Geometry check sheet. Reference: the model listing, model coordinates, mm. A direction names the side the tool comes from. Give positions to 0.01 mm unless a question says otherwise; leave off trailing zeros. Order: outer loops, then holes, each group sorted by start corner. A loop starts at its lowest first (then second) coordinate and runs counter-clockwise, first axis right, second up. Notation, with made-up numbers: M -3.75,50 L 13.25,50 A20 cw 13.25,58 Z; hole C 4,14.5 d8. An arc over 180 degrees is marked long. Answer as a JSON object with one key per item and string values. Group by question number.
from build123d import *

# Parameters (mm, degrees)
SKETCH7_R             = 4.411628617
SKETCH7_R_2           = 1.499999999
BOSS_EXTRUDE1_DEPTH   = 15
SKETCH7_R_3           = 4.404719082
BOSS_EXTRUDE1_2_DEPTH = 15
BOSS_EXTRUDE1_3_DEPTH = 15
BOSS_EXTRUDE1_4_DEPTH = 15
SKETCH8_R             = 3.5
CUT_EXTRUDE1_DEPTH    = 5
SKETCH9_R             = 3.5
BOSS_EXTRUDE9_DEPTH   = 5
SKETCH12_R            = 2.1
BOSS_EXTRUDE10_DEPTH  = 5
FILLET3_R             = 4
SKETCH13_W            = 20
SKETCH13_H            = 20
SKETCH13_R            = 2.383284349
BOSS_EXTRUDE11_DEPTH  = 5
FILLET4_R             = 4
SKETCH14_R            = 2.383284349
SKETCH14_R_2          = 2.1
SKETCH14_W            = 20
SKETCH14_H            = 40
BOSS_EXTRUDE12_DEPTH  = 5
FILLET5_R             = 4
SKETCH15_W            = 31.82070186
SKETCH15_H            = 40
SKETCH15_R            = 2.1
BOSS_EXTRUDE13_DEPTH  = 5
FILLET6_R             = 4
SKETCH16_R            = 3.5
SKETCH16_R_2          = 1.499999999
BOSS_EXTRUDE14_DEPTH  = 15
CUT_EXTRUDE3_DEPTH    = 15
SKETCH18_R            = 13.5
CUT_EXTRUDE6_DEPTH    = 21


with BuildPart() as part:
    # Sketch7 → Boss-Extrude1 (new body)
    with BuildSketch(Plane(origin=(0, 0, 0), x_dir=(1, 0, 0), z_dir=(0, 1, 0))):
        with Locations((-35.224970632, 25)):
            Circle(SKETCH7_R)
        with Locations((-35.224970632, 25)):
            Circle(SKETCH7_R_2, mode=Mode.SUBTRACT)
    extrude(amount=-BOSS_EXTRUDE1_DEPTH)


with BuildPart() as body_2:
    # Sketch7 → Boss-Extrude1 2 (new body)
    with BuildSketch(Plane(origin=(0, 0, 0), x_dir=(1, 0, 0), z_dir=(0, 1, 0))):
        with Locations((21.775029368, 31)):
            Circle(SKETCH7_R_3)
        with Locations((21.775029368, 31)):
            Circle(SKETCH7_R_2, mode=Mode.SUBTRACT)
    extrude(amount=-BOSS_EXTRUDE1_2_DEPTH)


with BuildPart() as body_3:
    # Sketch7 → Boss-Extrude1 3 (new body)
    with BuildSketch(Plane(origin=(0, 0, 0), x_dir=(1, 0, 0), z_dir=(0, 1, 0))):
        with Locations((21.775029368, -31)):
            Circle(SKETCH7_R_3)
        with Locations((21.775029368, -31)):
            Circle(SKETCH7_R_2, mode=Mode.SUBTRACT)
    extrude(amount=-BOSS_EXTRUDE1_3_DEPTH)


with BuildPart() as body_4:
    # Sketch7 → Boss-Extrude1 4 (new body)
    with BuildSketch(Plane(origin=(0, 0, 0), x_dir=(1, 0, 0), z_dir=(0, 1, 0))):
        with Locations((-35.224970632, -25)):
            Circle(SKETCH7_R)
        with Locations((-35.224970632, -25)):
            Circle(SKETCH7_R_2, mode=Mode.SUBTRACT)
    extrude(amount=-BOSS_EXTRUDE1_4_DEPTH)


with BuildPart() as cut_extrude1_tool:
    # Sketch8 → Cut-Extrude1 (new body)
    with BuildSketch(Plane(origin=(0, -15, 0), x_dir=(-1, 0, 0), z_dir=(0, -1, 0))):
        with Locations((35.224970632, -25)):
            Circle(SKETCH8_R)
        with Locations((-21.775029368, -31)):
            Circle(SKETCH8_R)
        with Locations((35.224970632, 25)):
            Circle(SKETCH8_R)
        with Locations((-21.775029368, 31)):
            Circle(SKETCH8_R)
    extrude(amount=-CUT_EXTRUDE1_DEPTH)


with BuildPart() as part_1:
    add(part.part)

    # Cut-Extrude1: cut by cut_extrude1_tool
    add(cut_extrude1_tool.part, mode=Mode.SUBTRACT)



with BuildPart() as body_2_1:
    add(body_2.part)

    # Cut-Extrude1: cut by cut_extrude1_tool
    add(cut_extrude1_tool.part, mode=Mode.SUBTRACT)


with BuildPart() as body_3_1:
    add(body_3.part)

    # Cut-Extrude1: cut by cut_extrude1_tool
    add(cut_extrude1_tool.part, mode=Mode.SUBTRACT)


with BuildPart() as body_4_1:
    add(body_4.part)

    # Cut-Extrude1: cut by cut_extrude1_tool
    add(cut_extrude1_tool.part, mode=Mode.SUBTRACT)


with BuildPart() as part_2:
    add(part_1.part)

    add(body_2_1.part)  # Boss-Extrude9 merges body 2

    add(body_3_1.part)  # Boss-Extrude9 merges body 3

    add(body_4_1.part)  # Boss-Extrude9 merges body 4
    # Sketch9 → Boss-Extrude9 (add)
    with BuildSketch(Plane(origin=(0, -15, 0), x_dir=(-1, 0, 0), z_dir=(0, -1, 0))):
        with BuildLine():
            Line((38.764660529, -27.633070923), (55.562895144, -8.838834765))
            ThreePointArc((55.562895144, -8.838834765), (59.224060379, 0), (55.562895144, 8.838834765))
            Line((55.562895144, 8.838834765), (38.764660529, 27.633070923))
            ThreePointArc((38.764660529, 27.633070923), (37.205669501, 28.941991761), (35.224970632, 29.411628617))
            Line((35.224970632, 29.411628617), (-20.858915448, 35.308397089))
            Line((-20.858915448, 35.308397089), (-21.775029368, 35.404719082))
            ThreePointArc((-21.775029368, 35.404719082), (-24.985189946, 34.016027065), (-26.171192213, 30.725587114))
            ThreePointArc((-26.171192213, 30.725587114), (-33.931933496, 0), (-26.171192213, -30.725587114))
            ThreePointArc((-26.171192213, -30.725587114), (-24.985189946, -34.016027065), (-21.775029368, -35.404719082))
            Line((-21.775029368, -35.404719082), (-20.858915448, -35.308397089))
            Line((-20.858915448, -35.308397089), (35.224970632, -29.411628617))
            ThreePointArc((35.224970632, -29.411628617), (37.205669501, -28.941991761), (38.764660529, -27.633070923))
        make_face()
        with Locations((-21.775029368, -31)):
            Circle(SKETCH9_R, mode=Mode.SUBTRACT)
        with Locations((35.224970632, -25)):
            Circle(SKETCH9_R, mode=Mode.SUBTRACT)
        with Locations((-21.775029368, 31)):
            Circle(SKETCH9_R, mode=Mode.SUBTRACT)
        with Locations((35.224970632, 25)):
            Circle(SKETCH9_R, mode=Mode.SUBTRACT)
    extrude(amount=BOSS_EXTRUDE9_DEPTH)

    # Sketch12 → Boss-Extrude10 (add)
    with BuildSketch(Plane(origin=(0, -15, 0), x_dir=(1, 0, 0), z_dir=(0, 1, 0))):
        Polygon((0, 29.508444845), (15.196340386, 29.508444845), (15.196340386, 44.508444845), (-20, 44.508444845), (-20, 29.508444845), (-15, 29.508444845), align=None)
        with Locations((-15, 39.200262185)):
            Circle(SKETCH12_R, mode=Mode.SUBTRACT)
        with Locations((10.196340386, 39.200262185)):
            Circle(SKETCH12_R, mode=Mode.SUBTRACT)
        Polygon((-20, -44.508444845), (-20, -29.508444845), (-15, -29.508444845), (0, -29.508444845), (15.196340386, -29.508444845), (15.196340386, -44.508444845), align=None)
        with Locations((-15, -39.200262185)):
            Circle(SKETCH12_R, mode=Mode.SUBTRACT)
        with Locations((10.196340386, -39.200262185)):
            Circle(SKETCH12_R, mode=Mode.SUBTRACT)
    extrude(amount=-BOSS_EXTRUDE10_DEPTH)

    # Fillet3
    fillet3_edges = [part_2.edges().sort_by_distance(p)[0] for p in [
        (15.196340386, -17.5, 44.508444845),
        (-20, -17.5, 44.508444845),
        (15.196340386, -17.5, -44.508444845),
        (-20, -17.5, -44.508444845),
    ]]
    fillet(fillet3_edges, radius=FILLET3_R)

    # Sketch13 → Boss-Extrude11 (add)
    with BuildSketch(Plane(origin=(0, -15, 0), x_dir=(1, 0, 0), z_dir=(0, 1, 0))):
        with Locations((-60.435748909, 0)):
            Rectangle(SKETCH13_W, SKETCH13_H)
        with Locations((-65.435748909, 5)):
            Circle(SKETCH13_R, mode=Mode.SUBTRACT)
        with Locations((-65.435748909, -5)):
            Circle(SKETCH13_R, mode=Mode.SUBTRACT)
    extrude(amount=-BOSS_EXTRUDE11_DEPTH)

    # Fillet4
    fillet4_edges = [part_2.edges().sort_by_distance(p)[0] for p in [
        (-70.435748909, -17.5, -10),
        (-70.435748909, -17.5, 10),
    ]]
    fillet(fillet4_edges, radius=FILLET4_R)

    # Sketch14 → Boss-Extrude12 (add)
    with BuildSketch(Plane(origin=(0, -15, 0), x_dir=(1, 0, 0), z_dir=(0, 1, 0))):
        with Locations((-65.435748909, 5)):
            Circle(SKETCH14_R)
        with Locations((-65.435748909, 5)):
            Circle(SKETCH14_R_2, mode=Mode.SUBTRACT)
        with Locations((-65.435748909, -5)):
            Circle(SKETCH14_R)
        with Locations((-65.435748909, -5)):
            Circle(SKETCH14_R_2, mode=Mode.SUBTRACT)
        with Locations((33.931933496, 0)):
            Rectangle(SKETCH14_W, SKETCH14_H)
        with Locations((38.931933496, 15)):
            Circle(SKETCH14_R_2, mode=Mode.SUBTRACT)
        with Locations((38.931933496, -15)):
            Circle(SKETCH14_R_2, mode=Mode.SUBTRACT)
    extrude(amount=-BOSS_EXTRUDE12_DEPTH)

    # Fillet5
    fillet5_edges = [part_2.edges().sort_by_distance(p)[0] for p in [
        (43.931933496, -17.5, -20),
        (43.931933496, -17.5, 20),
    ]]
    fillet(fillet5_edges, radius=FILLET5_R)

    # Sketch15 → Boss-Extrude13 (add)
    with BuildSketch(Plane(origin=(0, -15, 0), x_dir=(1, 0, 0), z_dir=(0, 1, 0))):
        with Locations((-54.525048972, 0)):
            Rectangle(SKETCH15_W, SKETCH15_H)
        with Locations((-65.435748909, 15)):
            Circle(SKETCH15_R, mode=Mode.SUBTRACT)
        with Locations((-65.435748909, -15)):
            Circle(SKETCH15_R, mode=Mode.SUBTRACT)
    extrude(amount=-BOSS_EXTRUDE13_DEPTH)

    # Fillet6
    fillet6_edges = [part_2.edges().sort_by_distance(p)[0] for p in [
        (-70.435399902, -17.5, -20),
        (-70.435399902, -17.5, 20),
    ]]
    fillet(fillet6_edges, radius=FILLET6_R)

    # Sketch16 → Boss-Extrude14 (add)
    with BuildSketch(Plane(origin=(0, -20, 0), x_dir=(-1, 0, 0), z_dir=(0, -1, 0))):
        with Locations((-21.775029368, -31)):
            Circle(SKETCH16_R)
        with Locations((-21.775029368, -31)):
            Circle(SKETCH16_R_2, mode=Mode.SUBTRACT)
        with Locations((-21.775029368, 31)):
            Circle(SKETCH16_R)
        with Locations((-21.775029368, 31)):
            Circle(SKETCH16_R_2, mode=Mode.SUBTRACT)
        with Locations((35.224970632, 25)):
            Circle(SKETCH16_R)
        with Locations((35.224970632, 25)):
            Circle(SKETCH16_R_2, mode=Mode.SUBTRACT)
        with Locations((35.224970632, -25)):
            Circle(SKETCH16_R)
        with Locations((35.224970632, -25)):
            Circle(SKETCH16_R_2, mode=Mode.SUBTRACT)
    extrude(amount=-BOSS_EXTRUDE14_DEPTH)

    # Sketch17 → Cut-Extrude3 (cut)
    with BuildSketch(Plane(origin=(0, -15, 0), x_dir=(1, 0, 0), z_dir=(0, 1, 0))):
        Polygon((-30.224970632, 15), (16.775029368, 20), (16.775029368, -20), (-30.224970632, -15), align=None)
    extrude(amount=-CUT_EXTRUDE3_DEPTH, mode=Mode.SUBTRACT)

    # Sketch18 → Cut-Extrude6 (cut, through all)
    with BuildSketch(Plane(origin=(0, 0, 0), x_dir=(1, 0, 0), z_dir=(0, 1, 0))):
        with Locations((-46.724970632, 0)):
            Circle(SKETCH18_R)
    extrude(amount=-CUT_EXTRUDE6_DEPTH, mode=Mode.SUBTRACT)


solid = part_2.part
1. Cross-section at C-C (z = -25). Record the cut outline in (x, y), and give its area (3 significant figures).
2. Cross-section at D-D (z = -9.5). Record the cut outline in (x, y), and give its area (3 significant figures).
3. Access from +Z, -Z, +X, -X, +Y, -Y to the whole of each face (thin tool, end or side, straight path). Record for faces 4 (the flat face through (-70.436, -17, 0)), 5 (the flat face through (-14, -15, 19)), 6 (the flat face through (43.932, -17, 0)), 7 (the flat face through (16.775, -17, 0)), 8 (the flat face through (-56, -17, -20)).
4. Thickness scan on line 1 along X through (y, z) = (-16.15, 0); line 2 along Z through (x, y) = (22, -4.75); line 3 along Z through (x, y) = (-15, -16). Record the ranges inside material, lowest first. Write a range as [from, to].
5. Cross-section at A-A (z = 0). Record the cut outline in (x, y), and give its area (3 significant figures).
6. Depth check by flat-ended pin: pin 1 (1 mm diameter, centred on x = 1, z = 26.5, fed in from +Y); pin 2 (5.5 mm diameter, centred on x = 38.93, z = 15, fed in from -Y); pin 3 (2.5 mm diameter, centred on x = -55, y = -18, fed in from -Z); pin 4 (5.5 mm diameter, centred on y = -16.5, z = 37.5, fed in from +X). Enter the tip coordinate at first touch or a pass-through.
7. Release check for a two-part mould opening along X. For faces 1 (the flat face through (35, -17, 20)), 2 (the cylindrical face through (-64.307, -17.465, 13.229)), 3 (the flat face through (-20, -17, 36)) record: released by +X, released by -X, zero draft, split by the parting line, or undercut.
8. Cross-section at B-B (y = -2). Record the cut outline in (x, z).
Report:
{
 "1": {"outline": "M -41.12,-20 L -36.72,-20 L -36.72,0 L -39.64,0 L -39.64,-15 L -41.12,-15 Z; M -33.72,-20 L 28.91,-20 L 28.91,-15 L -30.81,-15 L -30.81,0 L -33.72,0 Z", "area": "422 mm2"},
 "2": {"outline": "M -70.44,-20 L -56.32,-20 L -56.32,-15 L -70.44,-15 Z; M -37.13,-20 L -30.22,-20 L -30.22,-15 L -37.13,-15 Z; M 16.78,-20 L 43.93,-20 L 43.93,-15 L 16.78,-15 Z", "area": "241 mm2"},
 "3": {"face 4": "+Z, -Z, -X, +Y, -Y", "face 5": "+Y", "face 6": "+Z, -Z, +X, +Y, -Y", "face 7": "+Y, -Y", "face 8": "-Z, -X, +Y, -Y"},
 "4": {"line 1": "x = [-70.44, -60.22], [-33.22, -30.22], [16.78, 43.93]", "line 2": "z = [-35.4, -32.48], [-29.52, -26.6], [26.6, 29.52], [32.48, 35.4]", "line 3": "z = [-44.51, -41.3], [-37.1, -16.62], [16.62, 37.1], [41.3, 44.51]"},
 "5": {"outline": "M -70.44,-20 L -60.22,-20 L -60.22,-15 L -70.44,-15 Z; M -33.22,-20 L -30.22,-20 L -30.22,-15 L -33.22,-15 Z; M 16.78,-20 L 43.93,-20 L 43.93,-15 L 16.78,-15 Z", "area": "202 mm2"},
 "6": {"pin 1": "stops at y = -15", "pin 2": "stops at y = -20", "pin 3": "stops at z = -20", "pin 4": "stops at x = 24.09"},
 "7": {"face 1": "zero draft", "face 2": "undercut", "face 3": "released by -X"},
 "8": {"outline": "C -35.22,-25 d8.82; C -35.22,25 d8.82; C 21.78,-31 d8.81; C 21.78,31 d8.81; hole C -35.22,-25 d3; hole C -35.22,25 d3; hole C 21.78,-31 d3; hole C 21.78,31 d3"}
}
